Geometry: final body of the model. Coordinates: model frame, mm. A direction names the side the tool comes from. Round coordinates to 2 decimals unless told otherwise and drop trailing zeros. Loops run counter-clockwise (first coordinate to the right, second up) from the corner with the lowest first, then second, coordinate; pieces in that order, holes last. Notation, with made-up numbers: (-32.75, 0.5) - (19.25, 0.5) arc R17 cw to (19.25, 24.5) - close; hole circle Ø5 at (-5, 59.25). An arc over 180 degrees is marked (long way). Write item = value, one per line. Start each with the question number.
Item 1: First-contact query: pin 1 (5 mm diameter, centred on y = 6, z = -63.5, fed in from +X); pin 2 (1.5 mm diameter, centred on x = -2, y = 6.5, fed in from +Z); pin 3 (3 mm diameter, centred on x = -2, y = 6.5, fed in from +Z). Flat tips, straight axial feed; report the tip coordinate or a pass-through.
Item 2: Draft query along X for faces 1 (the cylindrical face through (-45.07, 5.601, -71.092)), 2 (the flat face through (50, 5, 70)), 3 (the flat face through (45, 2.5, 73)). Return one class per face: pulls with the +X half, pulls with the -X half, needs draft (parallel to the pull), parting line crosses it, or undercut.
Item 3: Section C-C (x = 36). Return loops of the section in (y, z).
Item 4: Line query: line 1 (Y direction, x = -46.75, z = -57); line 2 (X direction, y = 6.25, z = 68); line 3 (X direction, y = 2, z = -54.5). Output: solid intervals per line, ascending. Write a range as from..to.
Item 5: Section A-A (z = -65). Return loops of the section in (x, y), plus the area to 3 significant figures.
Item 6: Section D-D (z = 33.5). Return loops of the section in (x, y), plus the area to 4 significant figures.
Item 7: Access query for faces 4 (the flat face through (45, 5, 65)), 5 (the flat face through (-3, 10, 0)), 6 (the flat face through (-40, 2.7, -65.2)), 7 (the flat face through (40, 5, 70)), 8 (the flat face through (42, 5, 80)). Directions: +Z, -Z, +X, -X, +Y, -Y. A direction counts if a zero-diameter tool reaches every point of the face in a straight line with its end or side. Return the directions, or none.
Item 8: Section B-B (y = 5). Return loops of the section in (x, z).
Autodesk Inventor part; units mm, degrees
ref_plane "YZ Plane" through (0, 0, 0) normal (1, 0, 0) x (0, 1, 0)
ref_plane "XZ Plane" through (0, 0, 0) normal (0, 1, 0) x (-1, 0, 0)
ref_plane "XY Plane" through (0, 0, 0) normal (0, 0, 1) x (1, 0, 0)
sketch "Sketch1" plane through (0, 0, 0) normal (0, 1, 0) x (-1, 0, 0)
  line L0 (50, 80) -> (-50, 80) construction
  line L1 (-50, 80) -> (-50, -80) construction
  line L2 (-50, -80) -> (50, -80) construction
  line L3 (50, -80) -> (50, 80) construction
  line L4 (50, -80) -> (40, -80)
  line L5 (40, -80) -> (40, -50)
  line L6 (50, -80) -> (50, -50)
  line L7 (-50, 80) -> (-50, 60)
  line L8 (-50, 80) -> (-40, 80)
  line L9 (-40, 80) -> (-40, 60)
  line L10 (-40, 60) -> (50, -50)
  line L11 (-50, 60) -> (40, -50)
  point P0 (0, 0)
  point P1 (50, 0)
  point P2 (0, -80)
  dimension "d0" = 160
  dimension "d1" = 100
  dimension "d2" = 10
  dimension "d3" = 30
  dimension "d4" = 20
  dimension "d5" = 10
extrude "Extrusion1" add sketch "Sketch1" along normal blind 10
sketch "Sketch2" plane through (40, 0, 80) normal (0, 0, 1) x (1, 0, 0)
  line L0 (-90, 0) -> (0, 0) construction
  line L1 (10, 10) -> (-80, 10) construction
  line L2 (0, 0) -> (10, 10) construction
  line L3 (2.5, 7.5) -> (7.5, 7.5)
  line L4 (7.5, 7.5) -> (7.5, 2.5)
  line L5 (7.5, 2.5) -> (2.5, 2.5)
  line L6 (2.5, 2.5) -> (2.5, 7.5)
  line L7 (2.5, 7.5) -> (7.5, 2.5) construction
  line L8 (7.5, 7.5) -> (2.5, 2.5) construction
  point P0 (-40, 0)
  point P1 (5, 5)
  dimension "d8" = 5
  dimension "d9" = 5
extrude "Extrusion2" cut sketch "Sketch2" against normal blind 15
sketch "Sketch3" plane through (-50, 0, -80) normal (-1, 0, 0) x (0, 0, 1)
  line L0 (30, 0) -> (30, 10) construction
  line L1 (30, 5) -> (0, 5) construction
  line L2 (0, 0) -> (0, 10) construction
  line L3 (15, 5) -> (7, 5) construction
  line L4 (15, 5) -> (23, 5) construction
  circle A0 centre (7, 5) radius 2
  circle A1 centre (15, 5) radius 2
  circle A2 centre (23, 5) radius 2
  point P0 (80, 0)
  dimension "d12" = 8
  dimension "d13" = 8
  dimension "d14" = 4
  dimension "d15" = 4
  dimension "d16" = 4
extrude "Extrusion3" cut sketch "Sketch3" against normal blind 15
properties part number "Arm"
Taken from the geometry:
q1.pin_1 = -40
q1.pin_2 = 9.58
q1.pin_3 = 10.5
q2.face_1 = needs draft
q2.face_2 = pulls with the +X half
q2.face_3 = undercut
q3.outline = (0, 42.89) - (10, 42.89) - (10, 55.11) - (0, 55.11) - close
q4.line_1 = 0..3, 7..10
q4.line_2 = 40..42.5, 47.5..50
q4.line_3 = -50..-40
q5.outline = (-50, 0) - (-40, 0) - (-40, 3) - (-50, 3) - close; (-50, 7) - (-40, 7) - (-40, 10) - (-50, 10) - close
q5.area = 60.0 mm^2
q6.outline = (18.32, 0) - (28.32, 0) - (28.32, 10) - (18.32, 10) - close
q6.area = 100.0 mm^2
q7.face_4 = +Z
q7.face_5 = +Z, -Z, +X, -X, +Y
q7.face_6 = -Z, +X, +Y, -Y
q7.face_7 = +Z, -X, +Y, -Y
q7.face_8 = +Z, +X, -X, +Y, -Y
q8.outline = (-50, -80) - (-40, -80) - (-40, -75) - (-50, -75) - close; (-50, -71) - (-40, -71) - (-40, -67) - (-50, -67) - close; (-50, -63) - (-40, -63) - (-40, -59) - (-50, -59) - close; (-50, -55) - (-40, -55) - (-40, -50) - (50, 60) - (50, 80) - (47.5, 80) - (47.5, 65) - (42.5, 65) - (42.5, 80) - (40, 80) - (40, 60) - (-50, -50) - close
